Geometry check sheet. Reference: drawing and pictorial views, mm from the part's lowest x, y, z. A direction names the side the tool comes from. Give positions to 0.01 mm unless a question says otherwise; leave off trailing zeros. Order: outer loops, then holes, each group sorted by start corner. A loop starts at its lowest first (then second) coordinate and runs counter-clockwise, first axis right, second up. Notation, with made-up numbers: (-37.5, 77.5) -> (-20.5, 77.5) arc R22 ccw to (-20.5, 85.5) -> close; hole circle Ø3 at (55.5, 59.5). An arc over 180 degrees is marked (long way). Write each question's results on one line, items separated by ' | '.
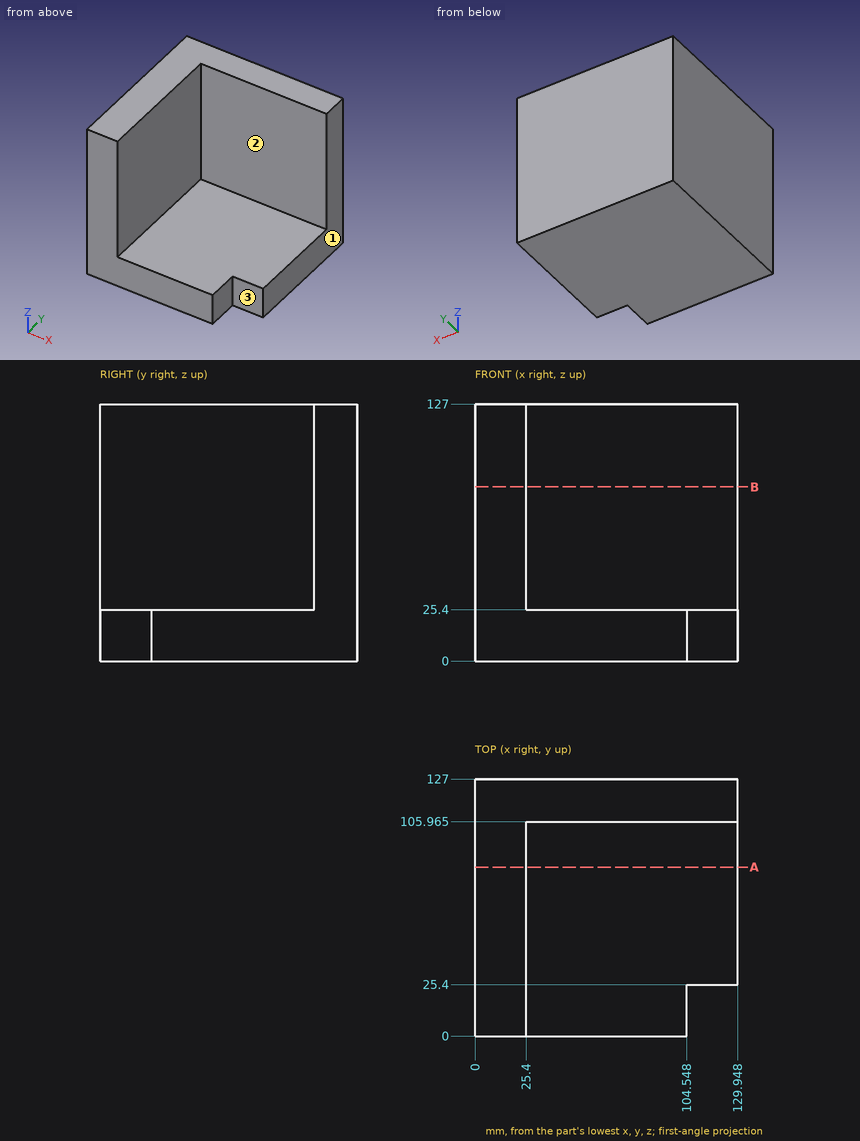
1. Section check B-B on z = 86. Record the cut outline in (x, y) (1 decimal), then the cut area to 4 significant figures.
Verdict:
outline: (0, 0) -> (25.4, 0) -> (25.4, 106) -> (129.9, 106) -> (129.9, 127) -> (0, 127) -> close | area: 5,425 mm^2
2. Section check A-A on y = 83.5. Record the cut outline in (x, z).
Verdict:
outline: (0, 0) -> (129.95, 0) -> (129.95, 25.4) -> (25.4, 25.4) -> (25.4, 127) -> (0, 127) -> close
3. Material ranges on probe 1 along Z at (x, y) = (85, 97); probe 2 along Y at (x, z) = (78, 74.5) (1 decimal), recorded low to high. Write a range as from..to.
Verdict:
probe 1: z = 0..25.4 | probe 2: y = 106..127
4. Access from +Z, -Z, +X, -X, +Y, -Y to the whole of each face (thin tool, end or side, straight path). Record for the marked faces 1, 2 and 3.
Verdict:
face 1: +Z, -Z, +X, +Y, -Y | face 2: +Z, +X, -Y | face 3: +Z, -Z, +X, -Y
5. Gauge pin test, flat ends, axial feed: pin 1 Ø12.5 at (x, z) = (116, 9) entering from -Y; pin 2 Ø3 at (y, z) = (55.5, 108.5) entering from +X; pin 3 Ø7.5 at (y, z) = (10.5, 11) entering from +X. Record the tip position at first contact, or that the pin passes through.
Verdict:
pin 1: stops at y = 25.4 | pin 2: stops at x = 25.4 | pin 3: stops at x = 104.55
